The listing builds one solid part. Answer for the finished solid, in the listing's coordinates (mm). A direction names the side the tool comes from. Coordinates: 2 decimals unless noted, no trailing zeros. Write each loop counter-clockwise with the first axis right and the second up, starting at its lowest first coordinate (ties: lowest second). Pieces come first, ordered by that corner, then holes.
from build123d import *

# Parameters (mm, degrees)
F0_W     = 104.771569
F0_H     = 75.58772
F1_DEPTH = 76.2
F2_W     = 84.611864
F2_H     = 50.140363
F3_DEPTH = 50.8
F4_W     = 25.4
F4_H     = 127
F5_DEPTH = 12.7
F6_W     = 25.4
F6_H     = 127
F7_DEPTH = 12.7


with BuildPart() as f1:
    # F0 (on Top) → F1 (new body)
    with BuildSketch(Plane.XY):
        with Locations((52.385784, 37.79386)):
            Rectangle(F0_W, F0_H)
    extrude(amount=F1_DEPTH)

    # F2 (on face) → F3 (cut)
    with BuildSketch(Plane.XY.offset(76.2)):
        with Locations((52.194364, 37.128242)):
            Rectangle(F2_W, F2_H)
    extrude(amount=-F3_DEPTH, mode=Mode.SUBTRACT)

    # F4 (on face) → F5 (join)
    with BuildSketch(Plane.XZ):
        with Locations((60.309702, 63.5)):
            Rectangle(F4_W, F4_H)
    extrude(amount=F5_DEPTH)

    # F6 (on face) → F7 (join)
    with BuildSketch(Plane(origin=(0, 75.58772, 0), x_dir=(-1, 0, 0), z_dir=(0, 1, 0))):
        with Locations((-54.248451, 63.5)):
            Rectangle(F6_W, F6_H)
    extrude(amount=F7_DEPTH)


solid = f1.part
1. A tool of negligible diameter and unlimited length cuts with its end or side. For faces 1 (the flat face through (52, 37, 25.4)), 2 (the flat face through (89, 0, 38)), 3 (the flat face through (23, 0, 38)), from which of +Z, -Z, +X, -X, +Y, -Y can it reach the whole face along a straight path? Write none if from no direction.
Results found:
face 1: +Z
face 2: +Z, -Z, +X, -Y
face 3: +Z, -Z, -X, -Y
2. Section D-D on x = 51 is taken. Give the vertices of the cut face in (y, z), then the cut area to 3 significant figures.
Results found:
outline: (-12.7, 0) - (88.29, 0) - (88.29, 127) - (75.59, 127) - (75.59, 76.2) - (62.2, 76.2) - (62.2, 25.4) - (12.06, 25.4) - (12.06, 76.2) - (0, 76.2) - (0, 127) - (-12.7, 127) - close
area: 6,440 mm2
3. Section A-A on x = 39 is taken. Give the vertices of the cut face in (y, z), then the cut area to 3 significant figures.
Results found:
outline: (0, 0) - (75.59, 0) - (75.59, 76.2) - (62.2, 76.2) - (62.2, 25.4) - (12.06, 25.4) - (12.06, 76.2) - (0, 76.2) - close
area: 3,210 mm2
4. Find the intervals of material crossed by L1, parallel to X at y = 24, z = 72.5; L2, parallel to Y at x = 94, z = 54.5; L3, parallel to Z at x = 10.5, y = 20, in increasing order.
Results found:
L1: x = 0 to 9.89, 94.5 to 104.77
L2: y = 0 to 12.06, 62.2 to 75.59
L3: z = 0 to 25.4
5. Flat-ended cylindrical pins translate along their axes: P1, Ø9.5, axis at x = 81.5, z = 41.5, coming from the -Y side; P2, Ø8, axis at y = 77.5, z = 94, coming from the -X side; P3, Ø10, axis at y = 85, z = 91.5, coming from the +X side; P4, Ø6, axis at x = 57.5, y = 77.5, coming from the -Z side. Find the tip coordinate at first contact, or state that the pin passes through.
Results found:
P1: stops at y = 0
P2: stops at x = 41.55
P3: stops at x = 66.95
P4: stops at z = 0
6. Section B-B on y = 24.5 is taken. Give the vertices of the cut face in (x, z), then the cut area to 3 significant figures.
Results found:
outline: (0, 0) - (104.77, 0) - (104.77, 76.2) - (94.5, 76.2) - (94.5, 25.4) - (9.89, 25.4) - (9.89, 76.2) - (0, 76.2) - close
area: 3,690 mm2
7. For a pull along Y with two mould halves and no side action, classify faces 4 (the flat face through (20, 75.588, 38)), 5 (the flat face through (66.948, 82, 63)), 6 (the flat face through (52, 12.058, 51)), 7 (the flat face through (60, 0, 102)) as pulls with the +Y half, pulls with the -Y half, needs draft (parallel to the pull), parting line crosses it, or undercut.
Results found:
face 4: pulls with the +Y half
face 5: needs draft
face 6: undercut
face 7: undercut
8. Section C-C on z = 23.5 is taken. Give the vertices of the cut face in (x, y), then the cut area to 3 significant figures.
Results found:
outline: (0, 0) - (47.61, 0) - (47.61, -12.7) - (73.01, -12.7) - (73.01, 0) - (104.77, 0) - (104.77, 75.59) - (66.95, 75.59) - (66.95, 88.29) - (41.55, 88.29) - (41.55, 75.59) - (0, 75.59) - close
area: 8,560 mm2
